Read the model definition and answer for the solid it produces. Units are mm, in the model's axes. Face numbers are marked on the shaded views. A direction names the side the tool comes from. Round coordinates to 2 decimals unless told otherwise and drop trailing zeros. Order: outer loops, then holes, each group sorted by start corner. A loop starts at its lowest first (then second) coordinate and runs counter-clockwise, first axis right, second up. Notation, with made-up numbers: (75.25, 41) - (134.25, 41) arc R20 ccw to (134.25, 52) - close; hole circle Ø4 at (87, -36.75). An arc over 180 degrees is marked (long way). Put each result on its own line as item: value. Start each with the question number.
Q1. This flat-tipped pin is pushed along its axis until it touches: pin 1 Ø4 at (x, y) = (132.5, 320) entering from +Z (3 decimals). Where does it stop, or does it pass through?
Q2. Section B-B on x = 25.4 is taken. Give the vertices of the cut face in (y, z) (3 decimals).
Q3. Section A-A on z = 25.4 is taken. Give the vertices of the cut face in (x, y) (3 decimals), then the cut area to 3 significant figures.
Q4. For a pull along X with two mould halves and no side action, classify the marked faces 3, 4 and 5 as pulls with the +X half, pulls with the -X half, needs draft (parallel to the pull), parting line crosses it, or undercut.
Q5. Section C-C on y = 287 is taken. Give the vertices of the cut face in (x, z) (3 decimals).
Q6. Which of the six approach directions +Z, -Z, +X, -X, +Y, -Y give full straight-line access (tool end or side, diameter ignored) to the marked faces 1 and 2?
Q7. Find the intervals of material crossed by line 1 along X through (y, z) = (1, 25); line 2 along Y through (x, z) = (353, 13.5) (3 decimals), in increasing order. Write a range as from..to.
from build123d import *

# Parameters (mm, degrees)
SKETCH1_W           = 381
SKETCH1_H           = 381
BOSS_EXTRUDE1_DEPTH = 50.8
SHELL1_T            = -3.175
SKETCH2_R           = 6.35
CUT_EXTRUDE1_DEPTH  = 417.576
SKETCH4_R           = 6.35
CUT_EXTRUDE2_DEPTH  = 417.576


with BuildPart() as part:
    # Sketch1 → Boss-Extrude1 (new body)
    with BuildSketch(Plane.XY):
        with Locations((190.5, 190.5)):
            Rectangle(SKETCH1_W, SKETCH1_H)
    extrude(amount=BOSS_EXTRUDE1_DEPTH)

    # Shell1
    shell1_openings = [part.faces().sort_by_distance(p)[0] for p in [
        (190.5, 190.5, 50.8),
    ]]
    offset(amount=SHELL1_T, openings=shell1_openings, kind=Kind.INTERSECTION)

    # Sketch2 → Cut-Extrude1 (cut)
    with BuildSketch(Plane(origin=(0, 381, 0), x_dir=(1, 0, 0), z_dir=(0, 1, 0))):
        with Locations(Location((25.4, -25.4, 0), (0, 0, 270))):
            Circle(SKETCH2_R)
    extrude(amount=-CUT_EXTRUDE1_DEPTH, mode=Mode.SUBTRACT)

    # Sketch4 → Cut-Extrude2 (cut)
    with BuildSketch(Plane(origin=(0, 381, 0), x_dir=(1, 0, 0), z_dir=(0, 1, 0))):
        with Locations((254, -25.4)):
            Circle(SKETCH4_R)
        with BuildLine():
            Line((254, -31.75), (355.6, -31.75))
            ThreePointArc((355.6, -31.75), (349.25, -25.4), (355.6, -19.05))
            Line((355.6, -19.05), (254, -19.05))
            ThreePointArc((254, -19.05), (258.490128061, -20.909871939), (260.35, -25.4))
            ThreePointArc((260.35, -25.4), (258.490128061, -29.890128061), (254, -31.75))
        make_face()
        with Locations((355.6, -25.4)):
            Circle(SKETCH4_R)
    extrude(amount=-CUT_EXTRUDE2_DEPTH, mode=Mode.SUBTRACT)


solid = part.part
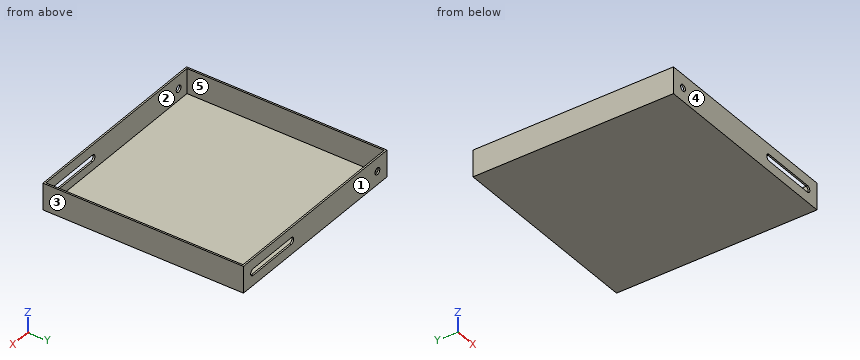
Findings:
1. pin 1: z = 3.175
2. outline: (0, 0) - (381, 0) - (381, 19.05) - (377.825, 19.05) - (377.825, 3.175) - (3.175, 3.175) - (3.175, 19.05) - (0, 19.05) - close; (0, 31.75) - (3.175, 31.75) - (3.175, 50.8) - (0, 50.8) - close; (377.825, 31.75) - (381, 31.75) - (381, 50.8) - (377.825, 50.8) - close
3. outline: (0, 0) - (19.05, 0) - (19.05, 3.175) - (3.175, 3.175) - (3.175, 377.825) - (19.05, 377.825) - (19.05, 381) - (0, 381) - close; (31.75, 0) - (247.65, 0) - (247.65, 3.175) - (31.75, 3.175) - close; (31.75, 377.825) - (247.65, 377.825) - (247.65, 381) - (31.75, 381) - close; (361.95, 0) - (381, 0) - (381, 381) - (361.95, 381) - (361.95, 377.825) - (377.825, 377.825) - (377.825, 3.175) - (361.95, 3.175) - close
3. area: 3,990 mm2
4. face 3: pulls with the +X half
4. face 4: needs draft
4. face 5: undercut
5. outline: (0, 0) - (381, 0) - (381, 50.8) - (377.825, 50.8) - (377.825, 3.175) - (3.175, 3.175) - (3.175, 50.8) - (0, 50.8) - close
6. face 1: +Z, -Z, +X, -X, +Y
6. face 2: +Z
7. line 1: 0..19.06, 31.74..247.66, 361.94..381
7. line 2: 0..3.175, 377.825..381
